Geometry check sheet. Reference: the model listing, model coordinates, mm. Round coordinates to 2 decimals unless told otherwise and drop trailing zeros. Order: outer loops, then holes, each group sorted by start corner. A loop starts at its lowest first (then second) coordinate and runs counter-clockwise, first axis right, second up. Notation, with made-up numbers: (63, -24) - (87, -24) arc R4 ccw to (87, -17) - close; hole circle Ø5 at (-1.5, 84). An arc over 180 degrees is marked (long way). Return JSON: item names as keys, results as strings. Group by question number.
Q1. Sectioned sample at C-C, the plane x = -37. Record the cut outline in (y, z).
Q2. Material ranges on line 1 along X through (y, z) = (0.6, 0); line 2 along Z through (x, y) = (-19.5, 0.6); line 3 along Z through (x, y) = (22, 0.7), recorded low to high.
Q3. Sectioned sample at D-D, the plane y = 0.45. Give the number of separate pieces and of enclosed holes in the cut face, then the cut area to 3 significant figures.
Q4. Sectioned sample at B-B, the plane z = -13. Record the cut outline in (x, y).
Q5. Sectioned sample at A-A, the plane x = 0. Record the cut outline in (y, z).
Q6. Gauge pin test, flat ends, axial feed: pin 1 Ø1.9 at (x, z) = (-32.04, -18.5) entering from -Y; pin 2 Ø0.9 at (x, y) = (80.5, 2) entering from +Z. Record the tip position at first contact, or that the pin passes through.
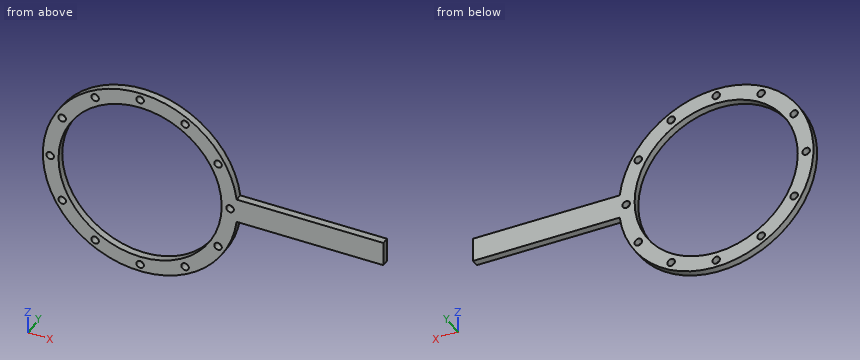
```python
from build123d import *

# Parameters (mm, degrees)
SKETCH1_R           = 40
SKETCH1_R_2         = 33.55
SKETCH1_W           = 60.313730334
SKETCH1_H           = 10
BOSS_EXTRUDE1_DEPTH = 3
SKETCH2_R           = 1.55
CUT_EXTRUDE1_DEPTH  = 108.745069493
CIRPATTERN1_COUNT   = 12


with BuildPart() as part:
    # Sketch1 → Boss-Extrude1 (new body)
    # profile 1 of 2: a face of its own
    with BuildSketch(Plane(origin=(0, 0, 0), x_dir=(1, 0, 0), z_dir=(0, 1, 0))):
        Circle(SKETCH1_R)
        with Locations(Location((0, 0, 0), (0, 0, 270))):
            Circle(SKETCH1_R_2, mode=Mode.SUBTRACT)
    # profile 2 of 2: a face of its own
    with BuildSketch(Plane(origin=(0, 0, 0), x_dir=(1, 0, 0), z_dir=(0, 1, 0))):
        with Locations((69.843134833, 0)):
            Rectangle(SKETCH1_W, SKETCH1_H)
    extrude(amount=BOSS_EXTRUDE1_DEPTH)

    # Sketch2 → Cut-Extrude1 (cut, through all)
    with BuildSketch(Plane(origin=(0, 3, 0), x_dir=(1, 0, 0), z_dir=(0, 1, 0))):
        with Locations(Location((37, 0, 0), (0, 0, 270))):
            Circle(SKETCH2_R)
    cut_extrude1 = extrude(amount=-CUT_EXTRUDE1_DEPTH, mode=Mode.SUBTRACT)

    # CirPattern1: Cut-Extrude1 ×12 about axis
    cirpattern1_axis = Axis((0, 0, 0), (0, 1, 0))
    for i in range(1, CIRPATTERN1_COUNT):
        add(cut_extrude1.rotate(cirpattern1_axis, i * 360 / CIRPATTERN1_COUNT), mode=Mode.SUBTRACT)


solid = part.part
```
Reply:
{
 "1": {"outline": "(0, -15.2) - (3, -15.2) - (3, -1.55) - (0, -1.55) - close; (0, 1.55) - (3, 1.55) - (3, 15.2) - (0, 15.2) - close"},
 "2": {"line 1": "-40 to -38.55, -35.45 to -33.55, 33.55 to 35.45, 38.55 to 100", "line 2": "-34.92 to -33.23, -30.86 to -27.3, 27.3 to 30.86, 33.23 to 34.92", "line 3": "-33.41 to -25.33, 25.33 to 33.41"},
 "3": {"separate pieces": "1", "enclosed holes": "13", "area": "2,000 mm^2"},
 "4": {"outline": "(-37.83, 0) - (-30.93, 0) - (-30.93, 3) - (-37.83, 3) - close; (30.93, 0) - (37.83, 0) - (37.83, 3) - (30.93, 3) - close"},
 "5": {"outline": "(0, -40) - (3, -40) - (3, -38.55) - (0, -38.55) - close; (0, -35.45) - (3, -35.45) - (3, -33.55) - (0, -33.55) - close; (0, 33.55) - (3, 33.55) - (3, 35.45) - (0, 35.45) - close; (0, 38.55) - (3, 38.55) - (3, 40) - (0, 40) - close"},
 "6": {"pin 1": "through", "pin 2": "z = 5"}
}
